The figure shows three views and two pictorial views of one solid part (mm, origin at its lowest corner). Answer the questions. Coordinates: 2 decimals unless noted, no trailing zeros. Order: outer loops, then holes, each group sorted by start corner. A loop starts at its lowest first (then second) coordinate and runs counter-clockwise, first axis right, second up. Notation, with made-up numbers: (24.25, 18) - (40.25, 18) arc R23 ccw to (40.25, 39) - close; hole circle Ø2 at (57.5, -20). An arc over 180 degrees is marked (long way). Use one line per item in the form item = value. Start each with the question number.
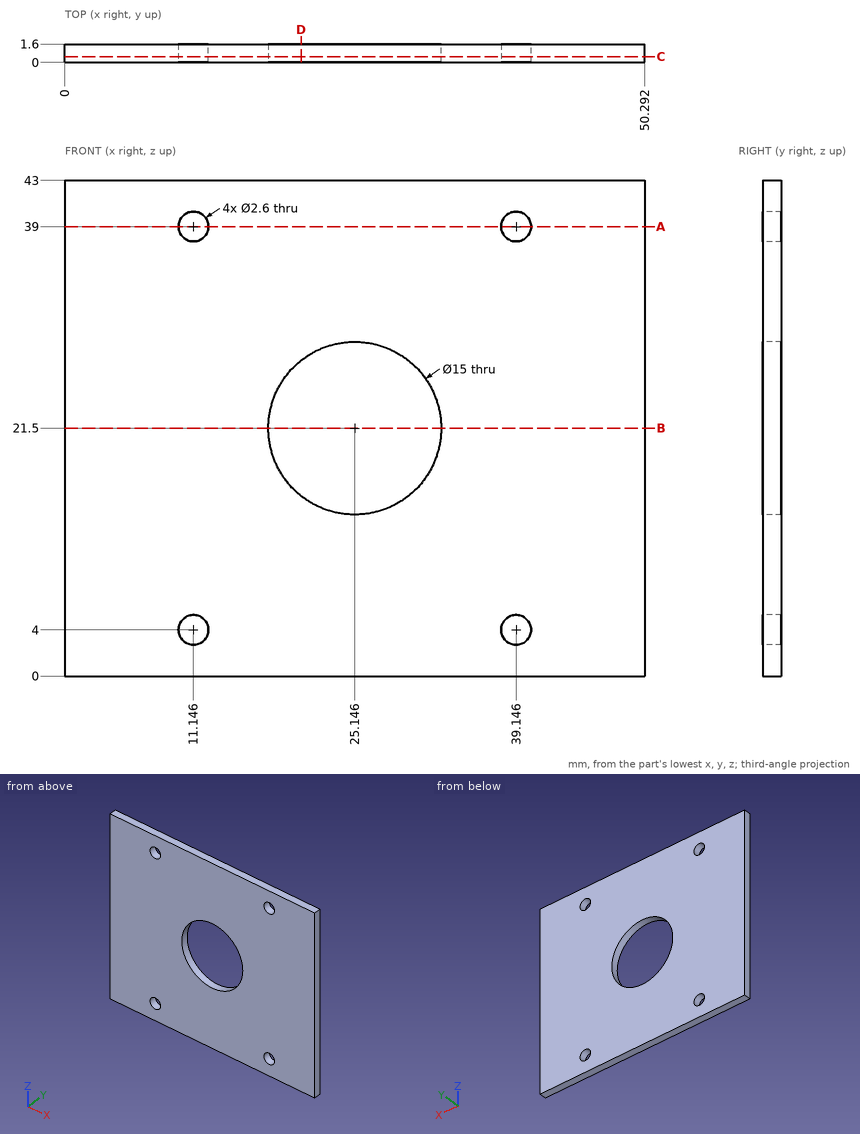
Q1. A cutting plane is placed at B-B (z = 21.5). Give the vertices of the cut face in (x, y).
Q2. Given P1, Ø2, axis at x = 11.146, z = 39, coming from the +Y side, flat-ended and moving along its own axis, determine where the tip first touches the part or whether it passes through.
Q3. A cutting plane is placed at A-A (z = 39). Give the vertices of the cut face in (x, y).
Q4. Consider probe 1 along X at (y, z) = (0.9, 39); probe 2 along X at (y, z) = (1.3, 38); probe 3 along Z at (x, y) = (25.5, 0.25). Determine where each line is inside the solid, lowest interval first.
Q5. A cutting plane is placed at C-C (y = 0.5). Give the vertices of the cut face in (x, z), then the cut area to 3 significant figures.
Q6. A cutting plane is placed at D-D (x = 20.5). Give the vertices of the cut face in (y, z), then the cut area to 3 significant figures.
Result sheet:
q1.outline = (0, 0) - (17.65, 0) - (17.65, 1.6) - (0, 1.6) - close; (32.65, 0) - (50.29, 0) - (50.29, 1.6) - (32.65, 1.6) - close
q2.P1 = through
q3.outline = (0, 0) - (9.85, 0) - (9.85, 1.6) - (0, 1.6) - close; (12.45, 0) - (37.85, 0) - (37.85, 1.6) - (12.45, 1.6) - close; (40.45, 0) - (50.29, 0) - (50.29, 1.6) - (40.45, 1.6) - close
q4.probe_1 = 0 to 9.85, 12.45 to 37.85, 40.45 to 50.29
q4.probe_2 = 0 to 10.32, 11.98 to 38.32, 39.98 to 50.29
q4.probe_3 = 0 to 14.01, 28.99 to 43
q5.outline = (0, 0) - (50.29, 0) - (50.29, 43) - (0, 43) - close; hole circle Ø2.6 at (11.15, 4); hole circle Ø2.6 at (11.15, 39); hole circle Ø15 at (25.15, 21.5); hole circle Ø2.6 at (39.15, 4); hole circle Ø2.6 at (39.15, 39)
q5.area = 1,960 mm^2
q6.outline = (0, 0) - (1.6, 0) - (1.6, 15.61) - (0, 15.61) - close; (0, 27.39) - (1.6, 27.39) - (1.6, 43) - (0, 43) - close
q6.area = 50.0 mm^2
